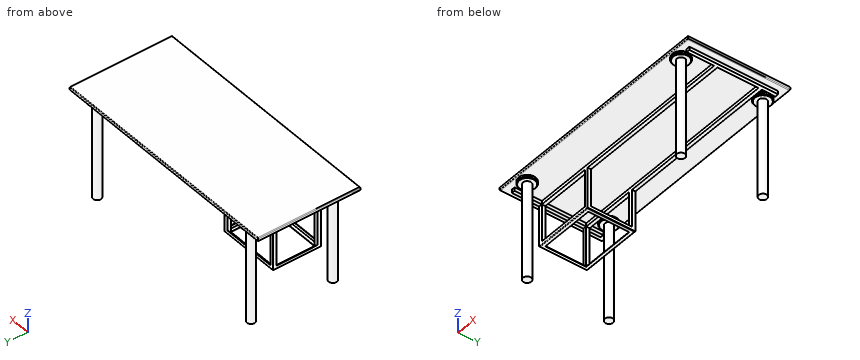
```python
from build123d import *

# Parameters (mm, degrees)
F0_W      = 1750
F0_H      = 750
F1_DEPTH  = 25
F2_W      = 1600
F2_H      = 300
F3_DEPTH  = 25
F4_R      = 62.5
F4_R_2    = 30
F5_DEPTH  = 20
F6_DEPTH  = 730
F7_W      = 25
F7_H      = 25
F8_DEPTH  = 300
F10_DEPTH = 300
F12_DEPTH = 400
F13_R     = 5
F14_R     = 5
F15_SIZE  = 5


with BuildPart() as f1:
    # F0 (on Top) → F1 (new body)
    with BuildSketch(Plane.XY):
        with Locations((101.9007265568, 24.7452616992)):
            Rectangle(F0_W, F0_H)
    extrude(amount=F1_DEPTH)

    # F2 (on face) → F3 (join)
    with BuildSketch(Plane(origin=(0, 0, 0), x_dir=(1, 0, 0), z_dir=(0, 0, -1))):
        Polygon((-698.0992734432, 300.2547383008), (-723.0992734432, 300.2547383008), (-723.0992734432, -324.7452616992), (-723.0992734432, -349.7452616992), (-698.0992734432, -349.7452616992), (-698.0992734432, -249.7452616992), (901.9007265568, -249.7452616992), (901.9007265568, -349.7452616992), (926.9007265568, -349.7452616992), (926.9007265568, -324.7452616992), (926.9007265568, 300.2547383008), (901.9007265568, 300.2547383008), (901.9007265568, 100.2547383008), (-698.0992734432, 100.2547383008), align=None)
        with Locations((101.9007265568, -74.7452616992)):
            Rectangle(F2_W, F2_H, mode=Mode.SUBTRACT)
    extrude(amount=F3_DEPTH)

    # F4 (on face) → F5 (join)
    with BuildSketch(Plane(origin=(0, 0, 0), x_dir=(1, 0, 0), z_dir=(0, 0, -1))):
        with Locations((816.9007265568, 275.2547383008)):
            Circle(F4_R)
        with Locations((816.9007265568, 275.2547383008)):
            Circle(F4_R_2, mode=Mode.SUBTRACT)
        with Locations((-613.0992734432, 275.2547383008)):
            Circle(F4_R)
        with Locations((-613.0992734432, 275.2547383008)):
            Circle(F4_R_2, mode=Mode.SUBTRACT)
        with Locations((-613.0992734432, -324.7452616992)):
            Circle(F4_R)
        with Locations((-613.0992734432, -324.7452616992)):
            Circle(F4_R_2, mode=Mode.SUBTRACT)
        with Locations((816.9007265568, -324.7452616992)):
            Circle(F4_R)
        with Locations((816.9007265568, -324.7452616992)):
            Circle(F4_R_2, mode=Mode.SUBTRACT)
    extrude(amount=F5_DEPTH)

    # F6 (add): faces of the model
    f6_faces = [f1.faces().sort_by_distance(p)[0] for p in [
        (816.9007265568, 324.7452616992, 0),
        (-613.0992734432, 324.7452616992, 0),
        (-613.0992734432, -275.2547383008, 0),
        (816.9007265568, -275.2547383008, 0),
    ]]
    extrude(f6_faces, amount=F6_DEPTH)

    # F7 (on face) → F8 (join)
    with BuildSketch(Plane(origin=(0, 0, -25), x_dir=(1, 0, 0), z_dir=(0, 0, -1))):
        with Locations((-710.5992734432, 87.7547383008)):
            Rectangle(F7_W, F7_H)
        with Locations((-285.5992734432, 87.7547383008)):
            Rectangle(F7_W, F7_H)
        with Locations((-285.5992734432, -237.2452616992)):
            Rectangle(F7_W, F7_H)
        with Locations((-710.5992734432, -237.2452616992)):
            Rectangle(F7_W, F7_H)
    extrude(amount=F8_DEPTH)

    # F9 (on face) → F10 (join, through all)
    with BuildSketch(Plane.XZ.offset(-224.7452616992)):
        Polygon((-723.0992734432, -300), (-723.0992734432, -325), (-720.0992734432, -325), (-719.87169981, -325), (-698.0992734432, -325), (-698.0992734432, -322), (-720.0992734432, -322), (-720.0992734432, -300), align=None)
        Polygon((-298.0992734432, -322), (-298.0992734432, -325), (-273.0992734432, -325), (-273.0992734432, -300), (-276.0992734432, -300), (-276.0992734432, -322), align=None)
    extrude(amount=F10_DEPTH)

    # F11 (on face) → F12 (join, through all)
    with BuildSketch(Plane(origin=(-298.0992734432, 0, 0), x_dir=(0, -1, 0), z_dir=(-1, 0, 0))):
        Polygon((-224.7452616992, -325), (-224.7452616992, -322), (-246.7452616992, -322), (-246.7452616992, -300), (-249.7452616992, -300), (-249.7452616992, -322), (-249.7452616992, -325), align=None)
        Polygon((97.2547383008, -322), (75.2547383008, -322), (75.2547383008, -325), (100.2547383008, -325), (100.2547383008, -322), (100.2547383008, -300), (97.2547383008, -300), align=None)
    extrude(amount=F12_DEPTH)

    # F13
    f13_edges = [f1.edges().sort_by_distance(p)[0] for p in [
        (-723.099273, 74.745262, -325),
        (-498.099273, -100.254738, -325),
        (-273.099273, 74.745262, -325),
        (-498.099273, 249.745262, -325),
    ]]
    fillet(f13_edges, radius=F13_R)

    # F14
    f14_edges = [f1.edges().sort_by_distance(p)[0] for p in [
        (101.900727, 399.745262, 25),
        (-773.099273, 24.745262, 25),
        (101.900727, -350.254738, 25),
        (976.900727, 24.745262, 25),
        (101.900727, -350.254738, 0),
        (-773.099273, 24.745262, 0),
        (976.900727, 24.745262, 0),
        (101.900727, 399.745262, 0),
    ]]
    fillet(f14_edges, radius=F14_R)

    # F15
    f15_edges = [f1.edges().sort_by_distance(p)[0] for p in [
        (-675.599273, -275.254738, -20),
        (754.400727, -275.254738, -20),
        (754.400727, 324.745262, -20),
        (-675.599273, 324.745262, -20),
    ]]
    chamfer(f15_edges, length=F15_SIZE)


solid = f1.part
```
Could you check a few things on this model? Use its own coordinates, in mm. Round coordinates to 2 decimals unless told otherwise and drop trailing zeros. Write each loop counter-clockwise with the first axis right and the second up, starting at its lowest first coordinate (ties: lowest second). Pieces come first, ordered by that corner, then holes.
(1) Suppose I cut it at D-D on x = 438. Write out the boundary of the cut face in (y, z).
Findings below:
outline: (-350.25, 5) arc R5 ccw to (-345.25, 0) - (-100.25, 0) - (-100.25, -25) - (-75.25, -25) - (-75.25, 0) - (224.75, 0) - (224.75, -25) - (249.75, -25) - (249.75, 0) - (394.75, 0) arc R5 ccw to (399.75, 5) - (399.75, 20) arc R5 ccw to (394.75, 25) - (-345.25, 25) arc R5 ccw to (-350.25, 20) - close
(2) If I drill on probe 1 along Z at (x, y) = (167, -294); probe 2 along X at (y, z) = (-294.5, -684); probe 3 along X at (y, z) = (299, -369), over which ranges is the centre line in solid material (lowest first)?
Findings below:
probe 1: z = 0 to 25
probe 2: x = -636.11 to -590.09, 793.89 to 839.91
probe 3: x = -628.5 to -597.7, 801.5 to 832.3
(3) Suppose I cut it at C-C on y = -174.5. Write out the boundary of the cut face in (x, z).
Findings below:
outline: (-773.1, 5) arc R5 ccw to (-768.1, 0) - (-723.1, 0) - (-723.1, -25) - (-698.1, -25) - (-698.1, 0) - (901.9, 0) - (901.9, -25) - (926.9, -25) - (926.9, 0) - (971.9, 0) arc R5 ccw to (976.9, 5) - (976.9, 20) arc R5 ccw to (971.9, 25) - (-768.1, 25) arc R5 ccw to (-773.1, 20) - close
(4) Suppose I cut it at A-A on x = -514.5. State how many separate pieces and enclosed holes the cut face has, and give its area (3 significant figures).
Findings below:
separate pieces: 3
enclosed holes: 0
area: 20,200 mm2
(5) For pin 1 (12.5 mm diameter, centred on x = -705, z = -247, fed in from +Y); pin 2 (1.5 mm diameter, centred on x = 23.5, y = 134.5, fed in from -Z); pin 3 (1.5 mm diameter, centred on y = 103.5, z = -323.5, fed in from +X), each with a flat end and sliding along its axis, tell me the tip position at first contact or that it passes through.
Findings below:
pin 1: stops at y = 249.75
pin 2: stops at z = 0
pin 3: stops at x = -273.92
